Could you check a few things on this model? Use its own coordinates, in mm. Face numbers are marked on the shaded views. A direction names the side the tool comes from. Give positions to 0.01 mm unless a question says otherwise; leave off trailing zeros. Order: outer loops, then holes, each group sorted by start corner. A loop starts at its lowest first (then second) coordinate and runs counter-clockwise, first axis right, second up. Notation, with made-up numbers: M 75.25,16 L 113.25,16 A17 cw 113.25,38 Z; hole C -12,-29.5 d11. An arc over 180 degrees is marked long. Use a Markdown table: item, result. Add a question column.
Item 1: Suppose I cut it at C-C on y = 5.25. Write out the boundary of the cut face in (x, z).
Item 2: I'm going to push flat-ended pins straight in: pin 1 Ø2.5 at (y, z) = (3.5, 4) entering from -X; pin 2 Ø3 at (x, z) = (5, 3) entering from -Y; pin 3 Ø1 at (x, z) = (11, 4) entering from -Y; pin 4 Ø4 at (x, y) = (2.52, 7.38) entering from +Z. Where does each tip first touch, or does it pass through?
Item 3: For the marked faces 4 and 5, which set-ups out of +Z, -Z, +X, -X, +Y, -Y let a thin tool reach every point of the face, with its end or its side?
Item 4: Suppose I cut it at A-A on z = 4.5. Write out the boundary of the cut face in (x, y).
Item 5: Suppose I cut it at D-D on y = 6.5. Write out the boundary of the cut face in (x, z), plus the area to 3 significant figures.
Item 6: If we mould it in two halves opening along Z, with no side actions, what happens to the marked faces 1, 2 and 3? For each: released by +Z, released by -Z, zero draft, split by the parting line, or undercut.
Item 7: Suppose I cut it at B-B on x = 14.25. Write out the boundary of the cut face in (y, z), plus the area to 3 significant figures.
Item 8: If I drill on L1, parallel to Z at x = 14.5, y = 7; L2, parallel to X at y = 0.75, z = 3.4; L3, parallel to Z at x = 12, y = 4.5, over which ranges is the centre line in solid material (lowest first)? Write a range as from..to.
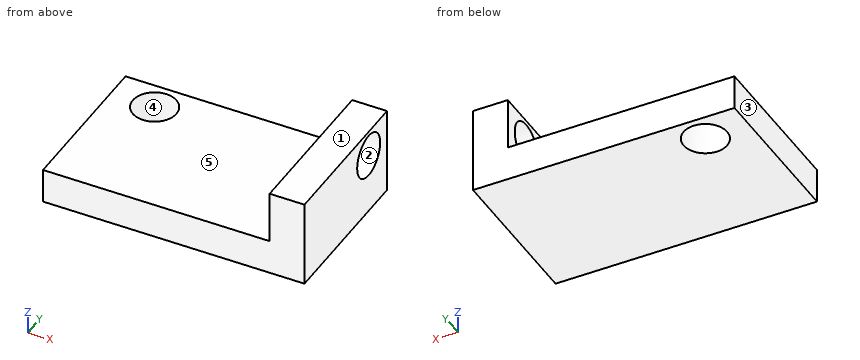
from build123d import *

# Parameters (mm, degrees)
F0_W     = 15
F0_H     = 9
F0_R     = 1.25
F2_DEPTH = 2
F1_W     = 2
F1_H     = 9
F3_DEPTH = 5
F4_R     = 1.25
F5_DEPTH = 25


with BuildPart() as f2:
    # F0 (on Top) → F2 (new body)
    with BuildSketch(Plane.XY):
        with Locations((7.5, 4.5)):
            Rectangle(F0_W, F0_H)
        with Locations((2.522875, 7.376701)):
            Circle(F0_R, mode=Mode.SUBTRACT)
    extrude(amount=F2_DEPTH)

    # F1 (on Top) → F3 (join)
    with BuildSketch(Plane.XY):
        with Locations((14, 4.5)):
            Rectangle(F1_W, F1_H)
    extrude(amount=F3_DEPTH)

    # F4 (on face) → F5 (cut)
    with BuildSketch(Plane(origin=(13, 0, 0), x_dir=(0, -1, 0), z_dir=(-1, 0, 0))):
        with Locations((-7, 3.5)):
            Circle(F4_R)
    extrude(amount=-F5_DEPTH, mode=Mode.SUBTRACT)


solid = f2.part
Findings below:
| question | item | result |
|---|---|---|
| 1 | outline | M 0,0 L 15,0 L 15,5 L 13,5 L 13,2 L 0,2 Z |
| 2 | pin 1 | stops at x = 13 |
| 2 | pin 2 | stops at y = 0 |
| 2 | pin 3 | passes through |
| 2 | pin 4 | stops at z = 2 |
| 3 | face 4 | +Z, -Z |
| 3 | face 5 | +Z, -X, +Y, -Y |
| 4 | outline | M 13,0 L 15,0 L 15,6.25 L 13,6.25 Z; M 13,7.75 L 15,7.75 L 15,9 L 13,9 Z |
| 5 | outline | M 0,0 L 1.63,0 L 1.63,2 L 0,2 Z; M 3.41,0 L 15,0 L 15,2.35 L 13,2.35 L 13,2 L 3.41,2 Z; M 13,4.65 L 15,4.65 L 15,5 L 13,5 Z |
| 5 | area | 27.9 mm^2 |
| 6 | face 1 | released by +Z |
| 6 | face 2 | undercut |
| 6 | face 3 | zero draft |
| 7 | outline | M 0,0 L 9,0 L 9,5 L 0,5 Z; hole C 7,3.5 d2.5 |
| 7 | area | 40.1 mm^2 |
| 8 | L1 | z = 0..2.25, 4.75..5 |
| 8 | L2 | x = 13..15 |
| 8 | L3 | z = 0..2 |
